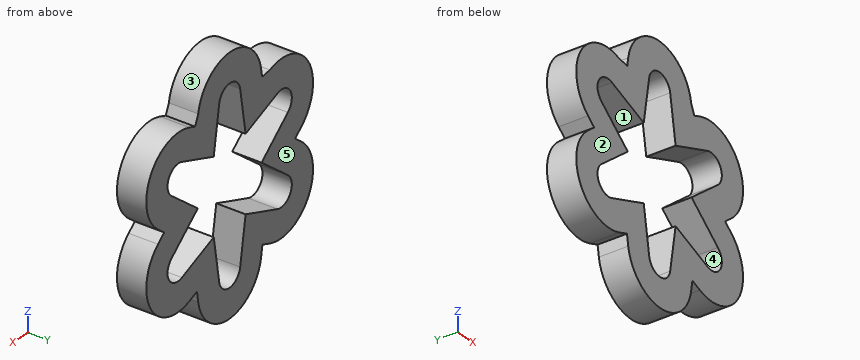
```python
from build123d import *

# Parameters (mm, degrees)
BOSS_EXTRUDE1_DEPTH = 5


with BuildPart() as part:
    # Sketch1 → Boss-Extrude1 (new body)
    with BuildSketch(Plane(origin=(0, 0, 0), x_dir=(1, 0, 0), z_dir=(0, 1, 0))):
        with BuildLine():
            Line((-9.463376853, 14.012074716), (-7.70451588, 13.344612952))
            Line((-7.70451588, 13.344612952), (-7.403124237, 15.201562119))
            ThreePointArc((-7.403124237, 15.201562119), (0, 21.5), (7.403124237, 15.201562119))
            Line((7.403124237, 15.201562119), (7.70451588, 13.344612952))
            Line((7.70451588, 13.344612952), (9.463376853, 14.012074716))
            ThreePointArc((9.463376853, 14.012074716), (18.619546181, 10.75), (16.866501091, 1.189487402))
            Line((16.866501091, 1.189487402), (15.40903176, 0))
            Line((15.40903176, 0), (16.866501091, -1.189487402))
            ThreePointArc((16.866501091, -1.189487402), (18.619546181, -10.75), (9.463376853, -14.012074716))
            Line((9.463376853, -14.012074716), (8.145790319, -13.512070085))
            Line((8.145790319, -13.512070085), (7.403124237, -15.201562119))
            ThreePointArc((7.403124237, -15.201562119), (0, -21.5), (-7.403124237, -15.201562119))
            Line((-7.403124237, -15.201562119), (-7.630525703, -13.800484906))
            Line((-7.630525703, -13.800484906), (-9.463376853, -14.012074716))
            ThreePointArc((-9.463376853, -14.012074716), (-18.619546181, -10.75), (-16.866501091, -1.189487402))
            Line((-16.866501091, -1.189487402), (-15.40903176, 0))
            Line((-15.40903176, 0), (-16.866501091, 1.189487402))
            ThreePointArc((-16.866501091, 1.189487402), (-18.619546181, 10.75), (-9.463376853, 14.012074716))
        make_face()
        with BuildLine():
            ThreePointArc((-11.23736272, 9.337358239), (-14.289419162, 8.25), (-13.705070799, 5.063162467))
            Line((-13.705070799, 5.063162467), (-7.504165125, 0.002404736))
            Line((-7.504165125, 0.002404736), (-7.504165125, -0.002404736))
            Line((-7.504165125, -0.002404736), (-13.705070799, -5.063162467))
            ThreePointArc((-13.705070799, -5.063162467), (-14.289419162, -8.25), (-11.23736272, -9.337358239))
            Line((-11.23736272, -9.337358239), (-3.754165125, -6.497595264))
            Line((-3.754165125, -6.497595264), (-3.75, -6.5))
            Line((-3.75, -6.5), (-2.467708079, -14.400520706))
            ThreePointArc((-2.467708079, -14.400520706), (0, -16.5), (2.467708079, -14.400520706))
            Line((2.467708079, -14.400520706), (3.75, -6.5))
            Line((3.75, -6.5), (3.754165125, -6.497595264))
            Line((3.754165125, -6.497595264), (11.23736272, -9.337358239))
            ThreePointArc((11.23736272, -9.337358239), (14.289419162, -8.25), (13.705070799, -5.063162467))
            Line((13.705070799, -5.063162467), (7.504165125, -0.002404736))
            Line((7.504165125, -0.002404736), (7.504165125, 0.002404736))
            Line((7.504165125, 0.002404736), (13.705070799, 5.063162467))
            ThreePointArc((13.705070799, 5.063162467), (14.289419162, 8.25), (11.23736272, 9.337358239))
            Line((11.23736272, 9.337358239), (3.754165125, 6.497595264))
            Line((3.754165125, 6.497595264), (3.75, 6.5))
            Line((3.75, 6.5), (2.467708079, 14.400520706))
            ThreePointArc((2.467708079, 14.400520706), (0, 16.5), (-2.467708079, 14.400520706))
            Line((-2.467708079, 14.400520706), (-3.75, 6.5))
            Line((-3.75, 6.5), (-3.754165125, 6.497595264))
            Line((-3.754165125, 6.497595264), (-11.23736272, 9.337358239))
        make_face(mode=Mode.SUBTRACT)
    extrude(amount=BOSS_EXTRUDE1_DEPTH)


solid = part.part
```
Verification items for the finished model (mm, model axes). Face numbers are marked on the shaded views. A direction names the side the tool comes from. Coordinates: 2 decimals unless noted, no trailing zeros. Loops run counter-clockwise (first coordinate to the right, second up) from the corner with the lowest first, then second, coordinate; pieces in that order, holes last. Notation, with made-up numbers: (67.5, -31) - (84.5, -31) arc R34 cw to (84.5, 0) - close; hole circle Ø2 at (-36.5, 71.25). An arc over 180 degrees is marked (long way). Return JSON: item names as keys, results as strings.
1. Thickness scan on L1, parallel to Z at x = 8.5, y = 2.9; L2, parallel to Z at x = 4, y = 4.05; L3, parallel to Z at x = 16, y = 0.9. Record the ranges inside material, lowest first.
Established:
{"L1": "z = -13.65 to -8.3, -0.82 to 0.82, 8.3 to 13.65", "L2": "z = -20.34 to -6.59, 6.59 to 20.34", "L3": "z = -13.42 to -0.48, 0.48 to 13.42"}
2. Section check B-B, the plane x = 6. Record the boundary of the cut face in (y, z), then the cut area to 3 significant figures.
Established:
{"outline": "(0, -18.5) - (5, -18.5) - (5, -7.35) - (0, -7.35) - close; (0, 7.35) - (5, 7.35) - (5, 18.5) - (0, 18.5) - close", "area": "112 mm2"}
3. Mould release check, pull along Z, two halves, no side actions. Record for the marked faces 3, 4 and 5: +Z half, -Z half, draft (parallel to the pull), parting line (faces both ways), or undercut.
Established:
{"face 3": "+Z half", "face 4": "undercut", "face 5": "draft"}
4. Go/stop test with flat-tipped pins: pin 1 (5 mm diameter, centred on x = -15, z = 5, fed in from -Y); pin 2 (1.5 mm diameter, centred on y = 1.5, z = 4, fed in from +X); pin 3 (3 mm diameter, centred on y = 1, z = -16.5, fed in from -X). Record where each tip stops, or that it passes through.
Established:
{"pin 1": "stops at y = 0", "pin 2": "stops at x = 19.28", "pin 3": "stops at x = -7.44"}
5. Section check A-A, the plane z = 0.5. Record the boundary of the cut face in (x, y).
Established:
{"outline": "(-16.02, 0) - (-8.11, 0) - (-8.11, 5) - (-16.02, 5) - close; (8.11, 0) - (16.02, 0) - (16.02, 5) - (8.11, 5) - close"}
6. Tool access check on the marked faces 1 and 2. Record the directions out of +Z, -Z, +X, -X, +Y, -Y that give a thin tool (end or side, any length) a straight path to the whole face; none if there is none.
Established:
{"face 1": "+Y, -Y", "face 2": "+Z, -Z, +X, -X, -Y"}
